Source: CAD feature listing. Evaluate the final solid. Frame: model axes, mm. A direction names the side the tool comes from. Coordinates: 2 decimals unless noted, no trailing zeros. Order: outer loops, then holes, each group sorted by start corner. A loop starts at its lowest first (then second) coordinate and runs counter-clockwise, first axis right, second up. Notation, with made-up numbers: (1, 50) - (27, 50) arc R20 ccw to (27, 82) - close; hole circle Ø7 at (35.5, -17.75). An arc over 180 degrees is marked (long way). One line per question, with ' | ' between items.
from build123d import *

# Parameters (mm, degrees)
EXTRUDE_1_DEPTH       = 82
FILLET_1_R            = 3
EXTRUDE_START         = -2
EXTRUDE_2_DEPTH       = 2
EXTRUDE_START_2       = -82
EXTRUDE_3_DEPTH       = 2
CUT_EXTRUDE_1_DEPTH   = 2
CUT_EXTRUDE_2_DEPTH   = 2
CUT_EXTRUDE_3_REACH   = 114.805
SKETCH_7_R            = 2
SKETCH_7_R_2          = 3.3
SKETCH_8_R            = 2
EXTRUDE_4_DEPTH       = 18
SKETCH_9_W            = 7
SKETCH_9_H            = 20
EXTRUDE_5_DEPTH       = 2
SKETCH_10_W           = 2
SKETCH_10_H           = 20
EXTRUDE_6_DEPTH       = 1
SKETCH_11_W           = 7
SKETCH_11_H           = 20
EXTRUDE_7_DEPTH       = 2
SKETCH_12_OUTSIDE_W   = 111.698
SKETCH_12_OUTSIDE_H   = 75.698
SKETCH_12_OUTSIDE_W_2 = 10
SKETCH_12_OUTSIDE_H_2 = 22
CUT_EXTRUDE_4_DEPTH   = 8
SKETCH_14_W           = 93.129876152
SKETCH_14_H           = 88.449918806
CUT_EXTRUDE_5_DEPTH   = 108.745069493


with BuildPart() as part:
    # Sketch 1 → Extrude 1 (new body)
    with BuildSketch(Plane.XY):
        Polygon((0, 0), (0, 2), (3, 2), (13, 12), (13, 37), (3, 47), (-60, 47), (-60, 49), (3, 49), (15, 37), (15, 12), (3, 0), align=None)
    extrude(amount=EXTRUDE_1_DEPTH)

    # Fillet 1
    fillet_1_edges = [part.edges().sort_by_distance(p)[0] for p in [
        (3, 2, 41),
        (13, 12, 41),
        (13, 37, 41),
        (3, 47, 41),
        (3, 49, 41),
        (15, 37, 41),
        (15, 12, 41),
        (3, 0, 41),
    ]]
    fillet(fillet_1_edges, radius=FILLET_1_R)

    # Sketch 4 → Extrude 2 (add)
    with BuildSketch(Plane(origin=(0, 0, 0), x_dir=(-1, 0, 0), z_dir=(0, 0, -1)).offset(EXTRUDE_START)):
        with BuildLine():
            Line((0, 0), (0, 26))
            Line((0, 26), (4, 26))
            Line((4, 26), (4, 27))
            Line((4, 27), (60, 27))
            Line((60, 27), (60, 49))
            Line((60, 49), (-1.757359313, 49))
            ThreePointArc((-1.757359313, 49), (-2.90540961, 48.771638598), (-3.878679656, 48.121320344))
            Line((-3.878679656, 48.121320344), (-14.121320344, 37.878679656))
            ThreePointArc((-14.121320344, 37.878679656), (-14.771638598, 36.90540961), (-15, 35.757359313))
            Line((-15, 35.757359313), (-15, 13.242640687))
            ThreePointArc((-15, 13.242640687), (-14.771638598, 12.09459039), (-14.121320344, 11.121320344))
            Line((-14.121320344, 11.121320344), (-3.878679656, 0.878679656))
            ThreePointArc((-3.878679656, 0.878679656), (-2.90540961, 0.228361402), (-1.757359313, 0))
            Line((-1.757359313, 0), (0, 0))
        make_face()
    extrude(amount=EXTRUDE_2_DEPTH)

    # Sketch 4_2 → Extrude 3 (add)
    with BuildSketch(Plane(origin=(0, 0, 0), x_dir=(-1, 0, 0), z_dir=(0, 0, -1)).offset(EXTRUDE_START_2)):
        with BuildLine():
            Line((0, 0), (0, 26))
            Line((0, 26), (4, 26))
            Line((4, 26), (4, 27))
            Line((4, 27), (60, 27))
            Line((60, 27), (60, 49))
            Line((60, 49), (-1.757359313, 49))
            ThreePointArc((-1.757359313, 49), (-2.90540961, 48.771638598), (-3.878679656, 48.121320344))
            Line((-3.878679656, 48.121320344), (-14.121320344, 37.878679656))
            ThreePointArc((-14.121320344, 37.878679656), (-14.771638598, 36.90540961), (-15, 35.757359313))
            Line((-15, 35.757359313), (-15, 13.242640687))
            ThreePointArc((-15, 13.242640687), (-14.771638598, 12.09459039), (-14.121320344, 11.121320344))
            Line((-14.121320344, 11.121320344), (-3.878679656, 0.878679656))
            ThreePointArc((-3.878679656, 0.878679656), (-2.90540961, 0.228361402), (-1.757359313, 0))
            Line((-1.757359313, 0), (0, 0))
        make_face()
    extrude(amount=EXTRUDE_3_DEPTH)

    # Sketch 5 → Cut-Extrude 1 (cut)
    with BuildSketch(Plane(origin=(0, 0, 0), x_dir=(-1, 0, 0), z_dir=(0, 0, -1))):
        Polygon((2.661599935, 45.0208), (2.661599935, 31), (0, 31), (0, 29.863095934), (55.9999896, 29.863095934), (55.9999896, 31), (53.469479015, 31), (53.469479015, 44.2999988), (37.469480535, 44.2999988), (37.469480535, 31), (36.113001155, 31), (36.113001155, 38.112), (19.512998795, 38.112), (19.512998795, 31), (17.861600015, 31), (17.861600015, 45.0208), align=None)
    extrude(amount=-CUT_EXTRUDE_1_DEPTH, mode=Mode.SUBTRACT)

    # Sketch 6 → Cut-Extrude 2 (cut)
    with BuildSketch(Plane.XY.offset(82)):
        Polygon((-55.9999896, 31), (-49.543385864, 31), (-49.543385864, 37.1214), (-33.143393264, 37.1214), (-33.143393264, 32.1214), (-29.143393264, 32.1214), (-29.143393264, 31), (-10.34416017, 31), (-10.34416017, 33.50000008), (-6.34416055, 33.50000008), (-6.34416055, 31), (0, 31), (0, 27), (0, 26), (-4, 26), (-4, 27), (-55.9999896, 27), align=None)
    extrude(amount=-CUT_EXTRUDE_2_DEPTH, mode=Mode.SUBTRACT)

    # Sketch 7 → Cut-Extrude 3 (cut, up to next)
    with BuildSketch(Plane(origin=(0, 49, 0), x_dir=(1, 0, 0), z_dir=(0, 1, 0)), mode=Mode.PRIVATE) as cut_extrude_3_sk1:
        with Locations((-52.4947896, -81.4948)):
            Circle(SKETCH_7_R)
    cut_extrude_3_tool1 = extrude(cut_extrude_3_sk1.sketch, amount=-CUT_EXTRUDE_3_REACH, mode=Mode.PRIVATE) & part.part
    # Sketch 7 → Cut-Extrude 3 (cut, up to next)
    with BuildSketch(Plane(origin=(0, 49, 0), x_dir=(1, 0, 0), z_dir=(0, 1, 0)), mode=Mode.PRIVATE) as cut_extrude_3_sk2:
        with Locations((-3.4981896, -81.4948)):
            Circle(SKETCH_7_R)
    cut_extrude_3_tool2 = extrude(cut_extrude_3_sk2.sketch, amount=-CUT_EXTRUDE_3_REACH, mode=Mode.PRIVATE) & part.part
    # Sketch 7 → Cut-Extrude 3 (cut, up to next)
    with BuildSketch(Plane(origin=(0, 49, 0), x_dir=(1, 0, 0), z_dir=(0, 1, 0)), mode=Mode.PRIVATE) as cut_extrude_3_sk3:
        with Locations(Location((-43.742640687, -20.5, 0), (0, 0, 180))):
            Circle(SKETCH_7_R_2)
    cut_extrude_3_tool3 = extrude(cut_extrude_3_sk3.sketch, amount=-CUT_EXTRUDE_3_REACH, mode=Mode.PRIVATE) & part.part
    # Sketch 7 → Cut-Extrude 3 (cut, up to next)
    with BuildSketch(Plane(origin=(0, 49, 0), x_dir=(1, 0, 0), z_dir=(0, 1, 0)), mode=Mode.PRIVATE) as cut_extrude_3_sk4:
        with Locations(Location((-2.742640687, -20.5, 0), (0, 0, 270))):
            Circle(SKETCH_7_R_2)
    cut_extrude_3_tool4 = extrude(cut_extrude_3_sk4.sketch, amount=-CUT_EXTRUDE_3_REACH, mode=Mode.PRIVATE) & part.part
    # Sketch 7 → Cut-Extrude 3 (cut, up to next)
    with BuildSketch(Plane(origin=(0, 49, 0), x_dir=(1, 0, 0), z_dir=(0, 1, 0)), mode=Mode.PRIVATE) as cut_extrude_3_sk5:
        with Locations(Location((-2.742640687, -61.5, 0), (0, 0, 180))):
            Circle(SKETCH_7_R_2)
    cut_extrude_3_tool5 = extrude(cut_extrude_3_sk5.sketch, amount=-CUT_EXTRUDE_3_REACH, mode=Mode.PRIVATE) & part.part
    # Sketch 7 → Cut-Extrude 3 (cut, up to next)
    with BuildSketch(Plane(origin=(0, 49, 0), x_dir=(1, 0, 0), z_dir=(0, 1, 0)), mode=Mode.PRIVATE) as cut_extrude_3_sk6:
        with Locations(Location((-43.742640687, -61.5, 0), (0, 0, 270))):
            Circle(SKETCH_7_R_2)
    cut_extrude_3_tool6 = extrude(cut_extrude_3_sk6.sketch, amount=-CUT_EXTRUDE_3_REACH, mode=Mode.PRIVATE) & part.part
    # Sketch 7 → Cut-Extrude 3 (cut, up to next)
    with BuildSketch(Plane(origin=(0, 49, 0), x_dir=(1, 0, 0), z_dir=(0, 1, 0)), mode=Mode.PRIVATE) as cut_extrude_3_sk7:
        with BuildLine():
            Line((-50, -66), (-50, -78))
            Line((-50, -78), (-53.9999896, -78))
            ThreePointArc((-53.9999896, -78), (-55.414203162, -78.585786438), (-55.9999896, -80))
            Line((-55.9999896, -80), (-60, -80))
            Line((-60, -80), (-60, -23.494789))
            ThreePointArc((-60, -23.494789), (-59.121320344, -25.616109344), (-57, -26.494789))
            Line((-57, -26.494789), (-52.436945771, -26.494789))
            ThreePointArc((-52.436945771, -26.494789), (-50.713764891, -27.208553891), (-50, -28.931734771))
            Line((-50, -28.931734771), (-50, -41))
            Line((-50, -41), (-50, -66))
        make_face()
    cut_extrude_3_tool7 = extrude(cut_extrude_3_sk7.sketch, amount=-CUT_EXTRUDE_3_REACH, mode=Mode.PRIVATE) & part.part
    # Sketch 7 → Cut-Extrude 3 (cut, up to next)
    with BuildSketch(Plane(origin=(0, 49, 0), x_dir=(1, 0, 0), z_dir=(0, 1, 0)), mode=Mode.PRIVATE) as cut_extrude_3_sk8:
        with BuildLine():
            Line((-38.742640687, -20.5), (-38.742640687, -16))
            Line((-38.742640687, -16), (-7.742640687, -16))
            Line((-7.742640687, -16), (-7.742640687, -20.5))
            ThreePointArc((-7.742640687, -20.5), (-6.278174593, -24.035533906), (-2.742640687, -25.5))
            Line((-2.742640687, -25.5), (1.757359313, -25.5))
            Line((1.757359313, -25.5), (1.757359313, -56.5))
            Line((1.757359313, -56.5), (-2.742640687, -56.5))
            ThreePointArc((-2.742640687, -56.5), (-6.278174593, -57.964466094), (-7.742640687, -61.5))
            Line((-7.742640687, -61.5), (-7.742640687, -66))
            Line((-7.742640687, -66), (-38.742640687, -66))
            Line((-38.742640687, -66), (-38.742640687, -61.5))
            ThreePointArc((-38.742640687, -61.5), (-40.207106781, -57.964466094), (-43.742640687, -56.5))
            Line((-43.742640687, -56.5), (-48.242640687, -56.5))
            Line((-48.242640687, -56.5), (-48.242640687, -25.5))
            Line((-48.242640687, -25.5), (-43.742640687, -25.5))
            ThreePointArc((-43.742640687, -25.5), (-40.207106781, -24.035533906), (-38.742640687, -20.5))
        make_face()
    cut_extrude_3_tool8 = extrude(cut_extrude_3_sk8.sketch, amount=-CUT_EXTRUDE_3_REACH, mode=Mode.PRIVATE) & part.part
    add(cut_extrude_3_tool1.solids().sort_by_distance((-52.49479, 49, 81.4948))[0], mode=Mode.SUBTRACT)
    add(cut_extrude_3_tool2.solids().sort_by_distance((-3.49819, 49, 81.4948))[0], mode=Mode.SUBTRACT)
    add(cut_extrude_3_tool3.solids().sort_by_distance((-43.742641, 49, 20.5))[0], mode=Mode.SUBTRACT)
    add(cut_extrude_3_tool4.solids().sort_by_distance((-2.742641, 49, 20.5))[0], mode=Mode.SUBTRACT)
    add(cut_extrude_3_tool5.solids().sort_by_distance((-2.742641, 49, 61.5))[0], mode=Mode.SUBTRACT)
    add(cut_extrude_3_tool6.solids().sort_by_distance((-43.742641, 49, 61.5))[0], mode=Mode.SUBTRACT)
    add(cut_extrude_3_tool7.solids().sort_by_distance((-55.073425, 49, 52.662221))[0], mode=Mode.SUBTRACT)
    add(cut_extrude_3_tool8.solids().sort_by_distance((-23.242641, 49, 41))[0], mode=Mode.SUBTRACT)

    # Sketch 8 → Extrude 4 (add)
    # profile 1 of 2: a face of its own
    with BuildSketch(Plane(origin=(0, 49, 0), x_dir=(1, 0, 0), z_dir=(0, 1, 0))):
        with BuildLine():
            Line((-6.34416055, -79), (0, -79))
            Line((0, -79), (0, -82))
            ThreePointArc((0, -82), (-0.878677535, -84.121318222), (-2.999994, -85))
            Line((-2.999994, -85), (-6.34416055, -85))
            Line((-6.34416055, -85), (-6.34416055, -82))
            Line((-6.34416055, -82), (-6.34416055, -79))
        make_face()
        with Locations(Location((-3.4981896, -81.4948, 0), (0, 0, 180))):
            Circle(SKETCH_8_R, mode=Mode.SUBTRACT)
    # profile 2 of 2: a face of its own
    with BuildSketch(Plane(origin=(0, 49, 0), x_dir=(1, 0, 0), z_dir=(0, 1, 0))):
        with BuildLine():
            Line((-49.543385864, -82), (-49.543385864, -79))
            Line((-49.543385864, -79), (-55.9999896, -79))
            Line((-55.9999896, -79), (-55.9999896, -82))
            ThreePointArc((-55.9999896, -82), (-55.121313822, -84.12131998), (-52.9999956, -85))
            Line((-52.9999956, -85), (-49.543385856, -85))
            Line((-49.543385856, -85), (-49.543385864, -82))
        make_face()
        with Locations(Location((-52.4947896, -81.4948, 0), (0, 0, 180))):
            Circle(SKETCH_8_R, mode=Mode.SUBTRACT)
    extrude(amount=-EXTRUDE_4_DEPTH)

    # Sketch 9 → Extrude 5 (add)
    with BuildSketch(Plane.ZY):
        with Locations((4.5, 11)):
            Rectangle(SKETCH_9_W, SKETCH_9_H)
        with Locations((77.5, 11)):
            Rectangle(SKETCH_9_W, SKETCH_9_H)
    extrude(amount=-EXTRUDE_5_DEPTH)

    # Sketch 10 → Extrude 6 (add)
    with BuildSketch(Plane.ZY):
        with Locations((7, 11)):
            Rectangle(SKETCH_10_W, SKETCH_10_H)
        with Locations((75, 11)):
            Rectangle(SKETCH_10_W, SKETCH_10_H)
    extrude(amount=EXTRUDE_6_DEPTH)

    # Sketch 11 → Extrude 7 (add)
    with BuildSketch(Plane.ZY.offset(1)):
        with Locations((4.5, 11)):
            Rectangle(SKETCH_11_W, SKETCH_11_H)
        with Locations((77.5, 11)):
            Rectangle(SKETCH_11_W, SKETCH_11_H)
    extrude(amount=EXTRUDE_7_DEPTH)

    # Sketch 12 outside → Cut-Extrude 4 (cut)
    with BuildSketch(Plane(origin=(15, 0, 0), x_dir=(0, 0, -1), z_dir=(1, 0, 0))):
        with Locations((-42.5, 24.5)):
            Rectangle(SKETCH_12_OUTSIDE_W, SKETCH_12_OUTSIDE_H)
        with Locations((-77, 11)):
            Rectangle(SKETCH_12_OUTSIDE_W_2, SKETCH_12_OUTSIDE_H_2, mode=Mode.SUBTRACT)
        with Locations((-5, 11)):
            Rectangle(SKETCH_12_OUTSIDE_W_2, SKETCH_12_OUTSIDE_H_2, mode=Mode.SUBTRACT)
    extrude(amount=-CUT_EXTRUDE_4_DEPTH, mode=Mode.SUBTRACT)

    # Sketch 14 → Cut-Extrude 5 (cut, through all)
    with BuildSketch(Plane(origin=(0, 21, 0), x_dir=(1, 0, 0), z_dir=(0, 1, 0))):
        with Locations((-39.564938076, -44.224959403)):
            Rectangle(SKETCH_14_W, SKETCH_14_H)
    extrude(amount=CUT_EXTRUDE_5_DEPTH, mode=Mode.SUBTRACT)


solid = part.part
(1) Cut plane C-C (z = 61). Return the cut outline in (x, y).
Taken from the geometry:
outline: (0, 0) - (1.76, 0) arc R3 ccw to (3.88, 0.88) - (7, 4) - (7, 6) - (3.88, 2.88) arc R3 cw to (1.76, 2) - (0, 2) - close
(2) Material intervals for L1, parallel to X at y = 16.5, z = 77; L2, parallel to Z at x = 10.25, y = 10.25; L3, parallel to Z at x = -0.5, y = 20, sorted ascending. Write a range as from..to.
Taken from the geometry:
L1: x = -3..-1, 0..2, 13..15 | L2: z = 0..2, 80..82 | L3: z = 6..8, 74..76
(3) Cut plane A-A (x = 10.5). Return the cut outline in (y, z), and give its area (3 significant figures).
Taken from the geometry:
outline: (7.5, 0) - (22, 0) - (22, 2) - (9.5, 2) - (9.5, 10) - (7.5, 10) - close; (7.5, 72) - (9.5, 72) - (9.5, 80) - (22, 80) - (22, 82) - (7.5, 82) - close | area: 90.0 mm²
(4) Pin query (flat end, axial travel): P1, Ø12, axis at y = 10, z = 44, coming from the -X side; P2, Ø0.9, axis at x = 1, z = 35.5, coming from the +Y side; P3, Ø0.8, axis at x = -0.5, y = 11.5, coming from the -Z side. Return the tip coordinate at first contact, or that it passes through.
Taken from the geometry:
P1: stops at x = 5 | P2: stops at y = 2 | P3: stops at z = 6
(5) Set-up query: faces 5 (the flat face through (-2, 1, 77)), 6 (the flat face through (-2, 11, 1)), 7 (the flat face through (7, 5, 41)), 8 (the cylindrical face through (12.765, 12.079, 76.056)), 9 (the flat face through (1, 2, 41)). Return all of +Z, -Z, +X, -X, +Y, -Y with unobstructed straight access to the full face (end or side cutting, diameter ignored); none if empty.
Taken from the geometry:
face 5: +Z, -Z, -X, -Y | face 6: -Z, -X, +Y, -Y | face 7: +X, +Y, -Y | face 8: +Y | face 9: -X, +Y
(6) Cut plane D-D (x = 6). Return the cut outline in (y, z), and give its area (3 significant figures).
Taken from the geometry:
outline: (3, 0) - (21, 0) - (21, 2) - (5, 2) - (5, 80) - (21, 80) - (21, 82) - (3, 82) - close | area: 228 mm²
(7) Pull-direction query (X, two-part tool) for faces 1 (the flat face through (-2, 11, 81)), 2 (the flat face through (8, 14, 80)), 3 (the flat face through (-3, 11, 4)), 4 (the cylindrical face through (14.78, 12.11, 5.07)); classes: pulls with the +X half, pulls with the -X half, needs draft (parallel to the pull), parting line crosses it, or undercut.
Taken from the geometry:
face 1: needs draft | face 2: undercut | face 3: pulls with the -X half | face 4: pulls with the +X half
(8) Cut plane B-B (y = 9). Return the cut outline in (x, z), and give its area (3 significant figures).
Taken from the geometry:
outline: (-3, 1) - (-1, 1) - (-1, 6) - (0, 6) - (0, 0) - (12, 0) - (12, 10) - (10, 10) - (10, 2) - (2, 2) - (2, 8) - (-3, 8) - close; (-3, 74) - (2, 74) - (2, 80) - (10, 80) - (10, 72) - (12, 72) - (12, 82) - (0, 82) - (0, 76) - (-1, 76) - (-1, 81) - (-3, 81) - close | area: 136 mm²
